Can you work these out from the model? Positions are in its coordinate system, mm. Round coordinates to 2 decimals unless told otherwise and drop trailing zeros. Loops run counter-clockwise (first coordinate to the right, second up) from the corner with the lowest first, then second, coordinate; pieces in that order, holes last.
(1) If I drill on line 1 along Z through (x, y) = (23.5, -0.35); line 2 along Z through (x, y) = (15, -0.15); line 3 along X through (y, z) = (-0.6, 22), over which ranges is the centre line in solid material (lowest first)?
(2) I want a section at A-A on z = -4. Write out the boundary of the cut face in (x, y).
(3) I want a section at B-B on x = 28.5. Write out the boundary of the cut face in (y, z), plus the area to 3 significant figures.
(4) Will these pins go through, and if not, where does the flat tip stop? pin 1 Ø6 at (x, z) = (-18.034, -18.034) entering from +Y; pin 2 Ø0.5 at (x, y) = (-14, -0.5) entering from -Z; pin 3 Ø0.5 at (y, z) = (-0.5, -14) entering from -X.
(5) Thinking about a two-plate mould opening in Z: for faces 1 (the face through (19.9, 0, -14.3)), 2 (the face through (15.518, -0.493, -21.885)), which applies, released by +Z, released by -Z, zero draft, split by the parting line, or undercut?
(6) I want a section at C-C on z = 24. Write out the boundary of the cut face in (x, y), plus the area to 3 significant figures.
(7) I want a section at D-D on x = -5.5. Write out the boundary of the cut face in (y, z), plus the area to 3 significant figures.
from build123d import *

# Parameters (mm, degrees)
F1_DEPTH = 1
F2_R     = 1.5875


with BuildPart() as f1:
    # F0 (on Front) → F1 (new body)
    with BuildSketch(Plane.XZ):
        with BuildLine():
            ThreePointArc((-18.034, 14.434), (-20.579584, 20.579584), (-14.434, 18.034))
            Line((-14.434, 18.034), (-13.434, 18.034))
            ThreePointArc((-13.434, 18.034), (-16.044953, 22.181733), (-20.913866, 21.620973))
            Line((-20.913866, 21.620973), (-31.14619, 31.853297))
            ThreePointArc((-31.14619, 31.853297), (-21.336036, 36.795638), (-10.427948, 35.499694))
            ThreePointArc((-10.427948, 35.499694), (-5.325882, 33.87639), (0, 33.3276))
            Line((0, 33.3276), (0, 34.3276))
            ThreePointArc((0, 34.3276), (-5.121964, 34.855377), (-10.02868, 36.416529))
            ThreePointArc((-10.02868, 36.416529), (-32.211491, 32.211491), (-36.416529, 10.02868))
            ThreePointArc((-36.416529, 10.02868), (-34.855377, 5.121964), (-34.3276, 0))
            Line((-34.3276, 0), (-33.3276, 0))
            ThreePointArc((-33.3276, 0), (-33.87639, 5.325882), (-35.499694, 10.427948))
            ThreePointArc((-35.499694, 10.427948), (-36.795638, 21.336036), (-31.853297, 31.14619))
            Line((-31.853297, 31.14619), (-21.620973, 20.913866))
            ThreePointArc((-21.620973, 20.913866), (-22.181733, 16.044953), (-18.034, 13.434))
            Line((-18.034, 13.434), (-18.034, 14.434))
        make_face()
    extrude(amount=F1_DEPTH)

    # F2
    f2_edges = [f1.edges().sort_by_distance(p)[0] for p in [
        (-31.853297, -0.5, 31.14619),
        (-31.14619, -0.5, 31.853297),
        (-20.913866, -0.5, 21.620973),
        (-21.620973, -0.5, 20.913866),
    ]]
    fillet(f2_edges, radius=F2_R)

    # F3: F1 across plane


with BuildPart() as f1_1:
    add(f1.part)
    add(f1.part.mirror(Plane.XY))

    # F4: F1 across plane


with BuildPart() as f1_2:
    add(f1_1.part)
    add(f1_1.part.mirror(Plane.YZ))


solid = f1_2.part
Filled sheet:
1. line 1: z = -37.32 to -36.28, -24.21 to -22.79, 22.79 to 24.21, 36.28 to 37.32
1. line 2: z = -37.85 to -36.84, -21.49 to -19.97, 19.97 to 21.49, 36.84 to 37.85
1. line 3: x = -37.69 to -36.67, -22.71 to -15.7, 15.7 to 22.71, 36.67 to 37.69
2. outline: (-34.65, -1) - (-33.64, -1) - (-33.64, 0) - (-34.65, 0) - close; (33.64, -1) - (34.65, -1) - (34.65, 0) - (33.64, 0) - close
3. outline: (-1, -35.14) - (0, -35.14) - (0, -33.95) - (-1, -33.95) - close; (-1, -29.21) - (0, -29.21) - (0, -27.79) - (-1, -27.79) - close; (-1, 27.79) - (0, 27.79) - (0, 29.21) - (-1, 29.21) - close; (-1, 33.95) - (0, 33.95) - (0, 35.14) - (-1, 35.14) - close
3. area: 5.20 mm2
4. pin 1: passes through
4. pin 2: stops at z = -37.72
4. pin 3: stops at x = -37.72
5. face 1: zero draft
5. face 2: undercut
6. outline: (-37.18, -1) - (-36.13, -1) - (-36.13, 0) - (-37.18, 0) - close; (-24.71, -1) - (-23.29, -1) - (-23.29, 0) - (-24.71, 0) - close; (23.29, -1) - (24.71, -1) - (24.71, 0) - (23.29, 0) - close; (36.13, -1) - (37.18, -1) - (37.18, 0) - (36.13, 0) - close
6. area: 4.93 mm2
7. outline: (-1, -34.94) - (0, -34.94) - (0, -33.91) - (-1, -33.91) - close; (-1, 33.91) - (0, 33.91) - (0, 34.94) - (-1, 34.94) - close
7. area: 2.05 mm2
